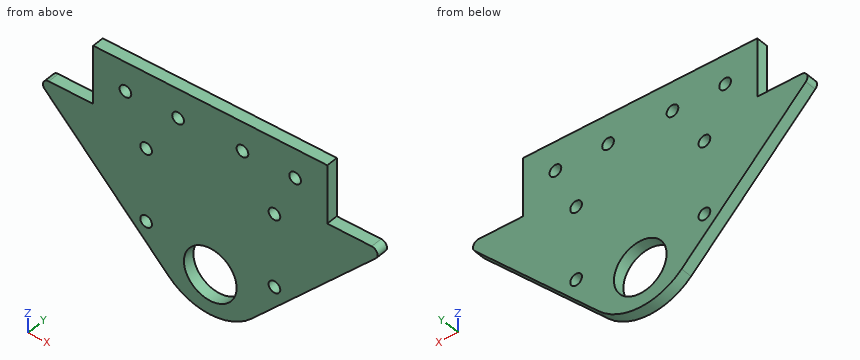
```python
from build123d import *

# Parameters (mm, degrees)
SKETCH_1_R      = 2.25
SKETCH_1_R_2    = 0.5
EXTRUDE_1_DEPTH = 1
FILLET_1_R      = 5
FILLET_3_R      = 0.5


with BuildPart() as part:
    # 草图1 → 凸台-拉伸1 (new body)
    with BuildSketch(Plane(origin=(0, 0, 0), x_dir=(1, 0, 0), z_dir=(0, 1, 0))):
        Polygon((-15, 0), (0, 15), (15, 0), (10, 0), (10, -5), (-10, -5), (-10, 0), align=None)
        with Locations(Location((0, 9.5, 0), (0, 0, 270))):
            Circle(SKETCH_1_R, mode=Mode.SUBTRACT)
        with Locations(Location((-5.482233047, 7.75, 0), (0, 0, 270))):
            Circle(SKETCH_1_R_2, mode=Mode.SUBTRACT)
        with Locations(Location((5.482233047, 7.75, 0), (0, 0, 90))):
            Circle(SKETCH_1_R_2, mode=Mode.SUBTRACT)
        with Locations(Location((-5.482233047, 1.5, 0), (0, 0, 270))):
            Circle(SKETCH_1_R_2, mode=Mode.SUBTRACT)
        with Locations(Location((5.482233047, 1.5, 0), (0, 0, 90))):
            Circle(SKETCH_1_R_2, mode=Mode.SUBTRACT)
        with Locations(Location((-7.25, -2.5, 0), (0, 0, 270))):
            Circle(SKETCH_1_R_2, mode=Mode.SUBTRACT)
        with Locations(Location((-2.75, -2.5, 0), (0, 0, 270))):
            Circle(SKETCH_1_R_2, mode=Mode.SUBTRACT)
        with Locations(Location((2.75, -2.5, 0), (0, 0, 90))):
            Circle(SKETCH_1_R_2, mode=Mode.SUBTRACT)
        with Locations(Location((7.25, -2.5, 0), (0, 0, 90))):
            Circle(SKETCH_1_R_2, mode=Mode.SUBTRACT)
    extrude(amount=EXTRUDE_1_DEPTH)

    # 圆角1
    fillet_1_edges = [part.edges().sort_by_distance(p)[0] for p in [
        (0, 0.5, -15),
    ]]
    fillet(fillet_1_edges, radius=FILLET_1_R)

    # 圆角3
    fillet_3_edges = [part.edges().sort_by_distance(p)[0] for p in [
        (-15, 0.5, 0),
        (15, 0.5, 0),
    ]]
    fillet(fillet_3_edges, radius=FILLET_3_R)


solid = part.part
```
The model under review builds one solid part; all positions refer to its coordinate system, in mm. Round coordinates to 2 decimals unless told otherwise and drop trailing zeros. Order: outer loops, then holes, each group sorted by start corner. A loop starts at its lowest first (then second) coordinate and runs counter-clockwise, first axis right, second up.
(1) Wall thickness on L1, parallel to X at y = 0.4, z = 2.5; L2, parallel to Z at x = 7.25, y = 0.4; L3, parallel to X at y = 0.65, z = -1.5: over which ranges is each line inside the solid? List them lowest first.
Working result:
L1: x = -10 to -7.75, -6.75 to -3.25, -2.25 to 2.25, 3.25 to 6.75, 7.75 to 10
L2: z = -7.75 to 2, 3 to 5
L3: x = -13.5 to -5.98, -4.98 to 4.98, 5.98 to 13.5
(2) Take a section at A-A, the plane z = -9.5. State the section outline as (x, y) points, plus the area to 3 significant figures.
Working result:
outline: (-5.5, 0) - (-2.25, 0) - (-2.25, 1) - (-5.5, 1) - close; (2.25, 0) - (5.5, 0) - (5.5, 1) - (2.25, 1) - close
area: 6.50 mm2
(3) Take a section at C-C, the plane z = 2.5. State the section outline as (x, y) points.
Working result:
outline: (-10, 0) - (-7.75, 0) - (-7.75, 1) - (-10, 1) - close; (-6.75, 0) - (-3.25, 0) - (-3.25, 1) - (-6.75, 1) - close; (-2.25, 0) - (2.25, 0) - (2.25, 1) - (-2.25, 1) - close; (3.25, 0) - (6.75, 0) - (6.75, 1) - (3.25, 1) - close; (7.75, 0) - (10, 0) - (10, 1) - (7.75, 1) - close
(4) Take a section at B-B, the plane x = -7.25. State the section outline as (y, z) points.
Working result:
outline: (0, -7.75) - (1, -7.75) - (1, 2) - (0, 2) - close; (0, 3) - (1, 3) - (1, 5) - (0, 5) - close
(5) For P1, Ø4, axis at x = 0, z = -9.5, coming from the +Y side, flat-tipped, find the tip position at first contact; note if it passes through.
Working result:
P1: passes through
(6) Take a section at D-D, the plane y = 0.85. Count the separate pieces of the cut face and the enclosed holes in it, plus the area to 3 significant figures.
Working result:
separate pieces: 1
enclosed holes: 9
area: 297 mm2
